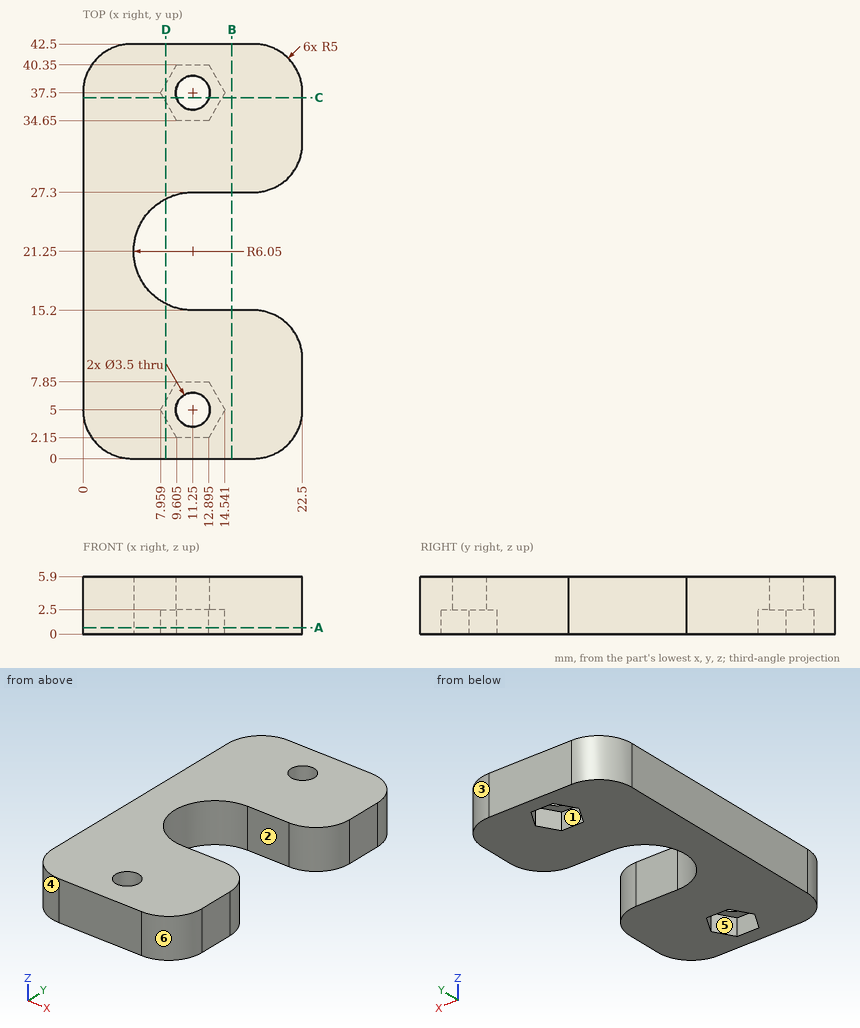
Could you check a few things on this drawing? It's one solid part, dimensions in mm from its lowest x, y, z. A direction names the side the tool comes from. Round coordinates to 2 decimals unless told otherwise and drop trailing zeros. Loops run counter-clockwise (first coordinate to the right, second up) from the corner with the lowest first, then second, coordinate; pieces in that order, holes last. Notation, with made-up numbers: M 13,8 L 69,8 A37 cw 69,45 Z; hole C 74,67 d10. An arc over 180 degrees is marked long. Write each question's results on one line, items separated by ' | '. Start each with the question number.
(1) I want a section at D-D (x = 8.5). Please give me the cut outline in (y, z).
(2) Will these pins go through, and if not, where does the flat tip stop? P1, Ø2, axis at x = 11.25, y = 5, coming from the +Z side; P2, Ø4.5, axis at x = 11.25, y = 37.5, coming from the -Z side; P3, Ø1, axis at x = 3, z = 3, coming from the -Y side.
(3) I want a section at C-C (y = 37). Please give me the cut outline in (x, z).
(4) I want a section at A-A (z = 0.65). State how many separate pieces and enclosed holes the cut face has, then the cut area to 3 significant figures.
(5) I want a section at B-B (x = 15.25). Please give me the cut outline in (y, z).
(6) Thinking about a two-plate mould opening in X: for the marked faces 4, 5 and 6, which applies, pulls with the +X half, pulls with the -X half, needs draft (parallel to the pull), parting line crosses it, or undercut?
(7) If I drill on probe 1 along Y at (x, z) = (11.25, 3.55); probe 2 along Y at (x, z) = (13.25, 5.5); probe 3 along X at (y, z) = (5, 4.9), over which ranges is the centre line in solid material (lowest first)? Write a range as from..to.
(8) On a 3-axis mill with a long thin cutter (end or side, diameter ignored), from which of +Z, -Z, +X, -X, +Y, -Y can I reach the whole of each face in a straight line? I mean the marked faces 1, 2 and 3. Say none if no direction works.
Solved:
1) outline: M 0,0 L 4.06,0 L 4.06,2.5 L 5.94,2.5 L 5.94,0 L 15.86,0 L 15.86,5.9 L 0,5.9 Z; M 26.64,0 L 36.56,0 L 36.56,2.5 L 38.44,2.5 L 38.44,0 L 42.5,0 L 42.5,5.9 L 26.64,5.9 Z
2) P1: passes through | P2: stops at z = 2.5 | P3: stops at y = 0.23
3) outline: M 0,0 L 8.25,0 L 8.25,2.5 L 9.57,2.5 L 9.57,5.9 L 0,5.9 Z; M 12.93,2.5 L 14.25,2.5 L 14.25,0 L 22.5,0 L 22.5,5.9 L 12.93,5.9 Z
4) separate pieces: 1 | enclosed holes: 2 | area: 674 mm²
5) outline: M 0,0 L 15.2,0 L 15.2,5.9 L 0,5.9 Z; M 27.3,0 L 42.5,0 L 42.5,5.9 L 27.3,5.9 Z
6) face 4: pulls with the -X half | face 5: undercut | face 6: pulls with the +X half
7) probe 1: y = 0..3.25, 6.75..15.2, 27.3..35.75, 39.25..42.5 | probe 2: y = 0..15.2, 27.3..42.5 | probe 3: x = 0..9.5, 13..22.5
8) face 1: -Z | face 2: +Z, -Z, +X | face 3: +Z, -Z, +X, +Y
